```python
from build123d import *

# Parameters (mm, degrees)
SKETCH1_R           = 60
BOSS_EXTRUDE1_DEPTH = 7
SKETCH2_W           = 10
SKETCH2_H           = 80
BOSS_EXTRUDE2_DEPTH = 163
SKETCH8_W           = 180
SKETCH8_H           = 50
BOSS_EXTRUDE5_DEPTH = 7
CHAMFER1_SIZE       = 2
CUT_EXTRUDE3_DEPTH  = 7
CUT_EXTRUDE4_REACH  = 9
SKETCH10_R          = 10
BOSS_EXTRUDE6_DEPTH = 3
SKETCH15_W          = 10
SKETCH15_H          = 80
CUT_EXTRUDE5_DEPTH  = 166
CUT_EXTRUDE6_REACH  = 9
CUT_EXTRUDE8_REACH  = 9
CUT_EXTRUDE9_REACH  = 9
SKETCH18_R          = 2
SKETCH19_W          = 180
SKETCH19_H          = 10
SKETCH19_W_2        = 32
SKETCH19_H_2        = 7
BOSS_EXTRUDE7_DEPTH = 7
CUT_EXTRUDE10_DEPTH = 10
CHAMFER2_SIZE       = 3
SKETCH21_W          = 15
SKETCH21_H          = 0.5
SKETCH22_R          = 16
SKETCH22_R_2        = 15
BOSS_EXTRUDE8_DEPTH = 1.5
SKETCH23_W          = 20
SKETCH23_H          = 60
BOSS_EXTRUDE9_DEPTH = 7
CHAMFER3_SIZE       = 2


with BuildPart() as part:
    # Sketch1 → Boss-Extrude1 (new body)
    with BuildSketch(Plane(origin=(0, 0, 0), x_dir=(1, 0, 0), z_dir=(0, 1, 0))):
        Circle(SKETCH1_R)
    extrude(amount=-BOSS_EXTRUDE1_DEPTH)

    # Sketch2 → Boss-Extrude2 (add)
    with BuildSketch(Plane(origin=(0, 0, 0), x_dir=(1, 0, 0), z_dir=(0, 1, 0))):
        with Locations((-33, 0)):
            Rectangle(SKETCH2_W, SKETCH2_H)
        with Locations((33, 0)):
            Rectangle(SKETCH2_W, SKETCH2_H)
    extrude(amount=BOSS_EXTRUDE2_DEPTH)

    # Sketch8 → Boss-Extrude5 (add)
    with BuildSketch(Plane(origin=(0, 0, 0), x_dir=(1, 0, 0), z_dir=(0, 1, 0))):
        with Locations((0, 30)):
            Rectangle(SKETCH8_W, SKETCH8_H)
    extrude(amount=-BOSS_EXTRUDE5_DEPTH)

    # Chamfer1
    chamfer1_edges = [part.edges().sort_by_distance(p)[0] for p in [
        (90, -3.5, -5),
        (-90, -3.5, -55),
        (90, -3.5, -55),
        (-90, -3.5, -5),
    ]]
    chamfer(chamfer1_edges, length=CHAMFER1_SIZE)

    # Sketch9 → Cut-Extrude3 (cut)
    with BuildSketch(Plane(origin=(0, 0, 0), x_dir=(1, 0, 0), z_dir=(0, 1, 0))):
        with BuildLine():
            Line((45, 33), (75, 33))
            ThreePointArc((75, 33), (78, 30), (75, 27))
            Line((75, 27), (45, 27))
            ThreePointArc((45, 27), (42, 30), (45, 33))
        make_face()
    cut_extrude3 = extrude(amount=-CUT_EXTRUDE3_DEPTH, mode=Mode.SUBTRACT)

    # Mirror4: Cut-Extrude3 across plane
    add(cut_extrude3.mirror(Plane(origin=(0, 0, 0), x_dir=(0, 0, 1), z_dir=(1, 0, 0))), mode=Mode.SUBTRACT)

    # Sketch10 → Cut-Extrude4 (cut, up to next)
    with BuildSketch(Plane(origin=(0, 0, 0), x_dir=(1, 0, 0), z_dir=(0, 1, 0)), mode=Mode.PRIVATE) as cut_extrude4_sk1:
        Circle(SKETCH10_R)
    cut_extrude4_tool1 = extrude(cut_extrude4_sk1.sketch, amount=-CUT_EXTRUDE4_REACH, mode=Mode.PRIVATE) & part.part
    add(cut_extrude4_tool1.solids().sort_by_distance((0, 0, 0))[0], mode=Mode.SUBTRACT)

    # Sketch12 → Cut-Revolve1 (revolve, cut)
    with BuildSketch(Plane.XY):
        Polygon((0, -7), (0, -3.5), (-14.5, -3.5), (-14.5, -3), (-21.5, -3), (-21.5, -3.5), (-21.5, -7), align=None)
    revolve(axis=Axis((0, -7, 0), (0, 1, 0)), mode=Mode.SUBTRACT)

    # Sketch14 → Boss-Extrude6 (add)
    with BuildSketch(Plane(origin=(0, 0, 0), x_dir=(1, 0, 0), z_dir=(0, 1, 0))):
        with BuildLine():
            ThreePointArc((8, 6), (0, 10), (-8, 6))
            Line((-8, 6), (8, 6))
        make_face()
    extrude(amount=-BOSS_EXTRUDE6_DEPTH)

    # Sketch15 → Cut-Extrude5 (cut)
    with BuildSketch(Plane(origin=(0, 163, 0), x_dir=(1, 0, 0), z_dir=(0, 1, 0))):
        with Locations((33, 0)):
            Rectangle(SKETCH15_W, SKETCH15_H)
        with Locations((-33, 0)):
            Rectangle(SKETCH15_W, SKETCH15_H)
    extrude(amount=-CUT_EXTRUDE5_DEPTH, mode=Mode.SUBTRACT)

    # Sketch16 → Cut-Extrude6 (cut, up to next)
    with BuildSketch(Plane(origin=(0, 0, 0), x_dir=(1, 0, 0), z_dir=(0, 1, 0)), mode=Mode.PRIVATE) as cut_extrude6_sk1:
        with BuildLine():
            Line((-51, -17), (-45, -17))
            ThreePointArc((-45, -17), (-42, -20), (-45, -23))
            Line((-45, -23), (-51, -23))
            ThreePointArc((-51, -23), (-54, -20), (-51, -17))
        make_face()
    cut_extrude6_tool1 = extrude(cut_extrude6_sk1.sketch, amount=-CUT_EXTRUDE6_REACH, mode=Mode.PRIVATE) & part.part
    add(cut_extrude6_tool1.solids().sort_by_distance((-48, 0, 20))[0], mode=Mode.SUBTRACT)
    # Sketch16 → Cut-Extrude6 (cut, up to next)
    with BuildSketch(Plane(origin=(0, 0, 0), x_dir=(1, 0, 0), z_dir=(0, 1, 0)), mode=Mode.PRIVATE) as cut_extrude6_sk2:
        with BuildLine():
            Line((51, -17), (45, -17))
            ThreePointArc((45, -17), (42, -20), (45, -23))
            Line((45, -23), (51, -23))
            ThreePointArc((51, -23), (54, -20), (51, -17))
        make_face()
    cut_extrude6_tool2 = extrude(cut_extrude6_sk2.sketch, amount=-CUT_EXTRUDE6_REACH, mode=Mode.PRIVATE) & part.part
    add(cut_extrude6_tool2.solids().sort_by_distance((48, 0, 20))[0], mode=Mode.SUBTRACT)

    # Sketch17 → Cut-Extrude8 (cut, up to next)
    with BuildSketch(Plane(origin=(0, 0, 0), x_dir=(1, 0, 0), z_dir=(0, 1, 0)), mode=Mode.PRIVATE) as cut_extrude8_sk1:
        with BuildLine():
            Line((-23, 33), (23, 33))
            ThreePointArc((23, 33), (26, 30), (23, 27))
            Line((23, 27), (-23, 27))
            ThreePointArc((-23, 27), (-26, 30), (-23, 33))
        make_face()
    cut_extrude8_tool1 = extrude(cut_extrude8_sk1.sketch, amount=-CUT_EXTRUDE8_REACH, mode=Mode.PRIVATE) & part.part
    add(cut_extrude8_tool1.solids().sort_by_distance((0, 0, -30))[0], mode=Mode.SUBTRACT)
    # Sketch17 → Cut-Extrude8 (cut, up to next)
    with BuildSketch(Plane(origin=(0, 0, 0), x_dir=(1, 0, 0), z_dir=(0, 1, 0)), mode=Mode.PRIVATE) as cut_extrude8_sk2:
        with BuildLine():
            Line((-15, -23), (-21, -23))
            ThreePointArc((-21, -23), (-24, -20), (-21, -17))
            Line((-21, -17), (-15, -17))
            ThreePointArc((-15, -17), (-12, -20), (-15, -23))
        make_face()
    cut_extrude8_tool2 = extrude(cut_extrude8_sk2.sketch, amount=-CUT_EXTRUDE8_REACH, mode=Mode.PRIVATE) & part.part
    add(cut_extrude8_tool2.solids().sort_by_distance((-18, 0, 20))[0], mode=Mode.SUBTRACT)
    # Sketch17 → Cut-Extrude8 (cut, up to next)
    with BuildSketch(Plane(origin=(0, 0, 0), x_dir=(1, 0, 0), z_dir=(0, 1, 0)), mode=Mode.PRIVATE) as cut_extrude8_sk3:
        with BuildLine():
            Line((15, -17), (21, -17))
            ThreePointArc((21, -17), (24, -20), (21, -23))
            Line((21, -23), (15, -23))
            ThreePointArc((15, -23), (12, -20), (15, -17))
        make_face()
    cut_extrude8_tool3 = extrude(cut_extrude8_sk3.sketch, amount=-CUT_EXTRUDE8_REACH, mode=Mode.PRIVATE) & part.part
    add(cut_extrude8_tool3.solids().sort_by_distance((18, 0, 20))[0], mode=Mode.SUBTRACT)

    # Sketch18 → Cut-Extrude9 (cut, up to next)
    with BuildSketch(Plane(origin=(0, 0, 0), x_dir=(1, 0, 0), z_dir=(0, 1, 0)), mode=Mode.PRIVATE) as cut_extrude9_sk1:
        with Locations((-46, 12.5)):
            Circle(SKETCH18_R)
    cut_extrude9_tool1 = extrude(cut_extrude9_sk1.sketch, amount=-CUT_EXTRUDE9_REACH, mode=Mode.PRIVATE) & part.part
    add(cut_extrude9_tool1.solids().sort_by_distance((-46, 0, -12.5))[0], mode=Mode.SUBTRACT)
    # Sketch18 → Cut-Extrude9 (cut, up to next)
    with BuildSketch(Plane(origin=(0, 0, 0), x_dir=(1, 0, 0), z_dir=(0, 1, 0)), mode=Mode.PRIVATE) as cut_extrude9_sk2:
        with Locations((-20, 12.5)):
            Circle(SKETCH18_R)
    cut_extrude9_tool2 = extrude(cut_extrude9_sk2.sketch, amount=-CUT_EXTRUDE9_REACH, mode=Mode.PRIVATE) & part.part
    add(cut_extrude9_tool2.solids().sort_by_distance((-20, 0, -12.5))[0], mode=Mode.SUBTRACT)
    # Sketch18 → Cut-Extrude9 (cut, up to next)
    with BuildSketch(Plane(origin=(0, 0, 0), x_dir=(1, 0, 0), z_dir=(0, 1, 0)), mode=Mode.PRIVATE) as cut_extrude9_sk3:
        with Locations((20, 12.5)):
            Circle(SKETCH18_R)
    cut_extrude9_tool3 = extrude(cut_extrude9_sk3.sketch, amount=-CUT_EXTRUDE9_REACH, mode=Mode.PRIVATE) & part.part
    add(cut_extrude9_tool3.solids().sort_by_distance((20, 0, -12.5))[0], mode=Mode.SUBTRACT)
    # Sketch18 → Cut-Extrude9 (cut, up to next)
    with BuildSketch(Plane(origin=(0, 0, 0), x_dir=(1, 0, 0), z_dir=(0, 1, 0)), mode=Mode.PRIVATE) as cut_extrude9_sk4:
        with Locations((46, 12.5)):
            Circle(SKETCH18_R)
    cut_extrude9_tool4 = extrude(cut_extrude9_sk4.sketch, amount=-CUT_EXTRUDE9_REACH, mode=Mode.PRIVATE) & part.part
    add(cut_extrude9_tool4.solids().sort_by_distance((46, 0, -12.5))[0], mode=Mode.SUBTRACT)

    # Sketch19 → Boss-Extrude7 (add)
    with BuildSketch(Plane(origin=(0, 0, 0), x_dir=(1, 0, 0), z_dir=(0, 1, 0))):
        with Locations((0, 55)):
            Rectangle(SKETCH19_W, SKETCH19_H)
        with Locations((74, 3.5)):
            Rectangle(SKETCH19_W_2, SKETCH19_H_2)
        with Locations((-74, 3.5)):
            Rectangle(SKETCH19_W_2, SKETCH19_H_2)
    extrude(amount=-BOSS_EXTRUDE7_DEPTH)

    # Sketch20 → Cut-Extrude10 (cut)
    with BuildSketch(Plane(origin=(0, 0, 0), x_dir=(1, 0, 0), z_dir=(0, 1, 0))):
        with BuildLine():
            ThreePointArc((68, 2), (66, 4), (68, 6))
            Line((68, 6), (78, 6))
            ThreePointArc((78, 6), (80, 4), (78, 2))
            Line((78, 2), (68, 2))
        make_face()
        with BuildLine():
            Line((78, 58), (68, 58))
            ThreePointArc((68, 58), (66, 56), (68, 54))
            Line((68, 54), (78, 54))
            ThreePointArc((78, 54), (80, 56), (78, 58))
        make_face()
        with BuildLine():
            ThreePointArc((-68, 58), (-66, 56), (-68, 54))
            Line((-68, 54), (-78, 54))
            ThreePointArc((-78, 54), (-80, 56), (-78, 58))
            Line((-78, 58), (-68, 58))
        make_face()
        with BuildLine():
            Line((-78, 2), (-68, 2))
            ThreePointArc((-68, 2), (-66, 4), (-68, 6))
            Line((-68, 6), (-78, 6))
            ThreePointArc((-78, 6), (-80, 4), (-78, 2))
        make_face()
    extrude(amount=-CUT_EXTRUDE10_DEPTH, mode=Mode.SUBTRACT)

    # Chamfer2
    chamfer2_edges = [part.edges().sort_by_distance(p)[0] for p in [
        (-90, -3.5, -60),
        (90, -3.5, -60),
        (90, -3.5, 0),
        (-90, -3.5, 0),
    ]]
    chamfer(chamfer2_edges, length=CHAMFER2_SIZE)

    # Sketch21 → Cut-Revolve2 (revolve, cut)
    with BuildSketch(Plane(origin=(0, 0, 0), x_dir=(0, 0, -1), z_dir=(1, 0, 0))):
        with Locations((7.5, -3.25)):
            Rectangle(SKETCH21_W, SKETCH21_H)
    revolve(axis=Axis((0, 0, 0), (0, -1, 0)), mode=Mode.SUBTRACT)

    # Sketch22 → Boss-Extrude8 (add)
    with BuildSketch(Plane.XZ.offset(3)):
        Circle(SKETCH22_R)
        Circle(SKETCH22_R_2, mode=Mode.SUBTRACT)
    extrude(amount=BOSS_EXTRUDE8_DEPTH)

    # Sketch23 → Boss-Extrude9 (add)
    with BuildSketch(Plane(origin=(0, 0, 0), x_dir=(1, 0, 0), z_dir=(0, 1, 0))):
        with Locations((-97, 30)):
            Rectangle(SKETCH23_W, SKETCH23_H)
        with Locations((97, 30)):
            Rectangle(SKETCH23_W, SKETCH23_H)
    extrude(amount=-BOSS_EXTRUDE9_DEPTH)

    # Chamfer3
    chamfer3_edges = [part.edges().sort_by_distance(p)[0] for p in [
        (-107, -3.5, 0),
        (-107, -3.5, -60),
        (107, -3.5, -60),
        (107, -3.5, 0),
    ]]
    chamfer(chamfer3_edges, length=CHAMFER3_SIZE)


solid = part.part
```
Model file for the job. Use its own axes, mm. A direction names the side the tool comes from. Round coordinates to 2 decimals unless told otherwise and drop trailing zeros. Write each loop counter-clockwise with the first axis right and the second up, starting at its lowest first coordinate (ties: lowest second). Pieces come first, ordered by that corner, then holes. Notation, with made-up numbers: (49.5, -9) - (98.5, -9) arc R19 ccw to (98.5, 26) - close; hole circle Ø3 at (28, 56.5). An arc over 180 degrees is marked (long way). One line per item, written item: value.
(1) Drop flat-ended pins along their axis: P1, Ø2, axis at x = -70.5, y = -2, coming from the +Z side; P2, Ø2.5, axis at x = -20, z = -12.5, coming from the -Y side; P3, Ø2.5, axis at x = 2, y = -1, coming from the +Z side; P4, Ø3, axis at x = -31, z = 9.5, coming from the +Y side. Give the stop position or say it passes through.
Values follow:
P1: stops at z = 0
P2: passes through
P3: stops at z = 60
P4: stops at y = -3
(2) 3-axis set-ups, long thin cutter, end or side, ignore diameter. For faces 3 (the flat face through (-18, -3, 17)), 4 (the flat face through (0, -3, -7)): which of +Z, -Z, +X, -X, +Y, -Y reach the whole face in a straight line?
Values follow:
face 3: +Y, -Y
face 4: -Y
(3) Cut at D-D, the plane z = 50.5. Give the cut face in (x, y).
Values follow:
outline: (-32.4, -7) - (32.4, -7) - (32.4, 0) - (-32.4, 0) - close
(4) Two-plate mould, pull along X, no slides. Class faces 1 (the flat face through (-1, 0, -14)), 2 (the cylindrical face through (80, -3, -4)): pulls with the +X half, pulls with the -X half, needs draft (parallel to the pull), parting line crosses it, or undercut.
Values follow:
face 1: needs draft
face 2: undercut
(5) Wall check: probe 1 along Z at (x, y) = (0, -3.7); probe 2 along Z at (x, y) = (-46, -5); probe 3 along Z at (x, y) = (-0.5, -6). Give the ranges that are in metal, low to high.
Values follow:
probe 1: z = -60 to -33, -27 to -21.5, -16 to -15, 15 to 16, 21.5 to 60
probe 2: z = -60 to -33, -27 to -14.5, -10.5 to 17, 23 to 38.52
probe 3: z = -60 to -33, -27 to -21.49, 21.49 to 60
(6) Cut at B-B, the plane x = -89.5. Give the cut face in (y, z).
Values follow:
outline: (-7, -60) - (0, -60) - (0, 0) - (-7, 0) - close
(7) Cut at A-A, the plane z = 19.5. Give the number of separate pieces and of enclosed holes in the cut face, plus the area to 3 significant figures.
Values follow:
separate pieces: 5
enclosed holes: 0
area: 328 mm²
